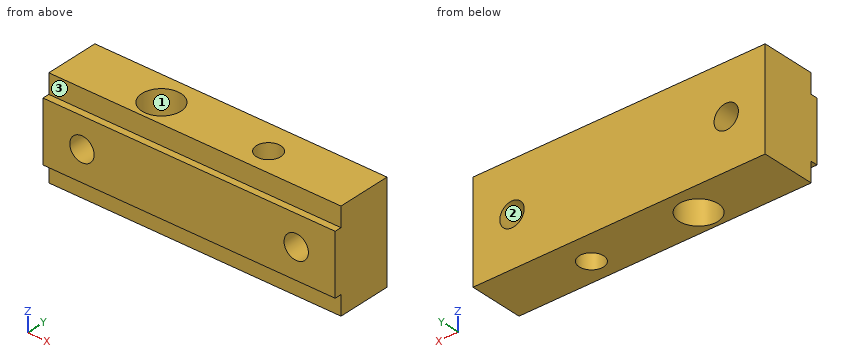
```python
from build123d import *

# Parameters (mm, degrees)
SKETCH1_W                  = 30
SKETCH1_H                  = 10.2
BOSS_EXTRUDE1_DEPTH        = 6.25
F_4_0_4_DIAMETER_HOLE1_D   = 4
F_2_5_2_5_DIAMETER_HOLE2_D = 2.5
F_2_5_2_5_DIAMETER_HOLE1_D = 2.5
SKETCH6_W                  = 2
SKETCH6_H                  = 0.7
CUT_EXTRUDE1_DEPTH         = 31


with BuildPart() as part:
    # Sketch1 → Boss-Extrude1 (new body)
    with BuildSketch(Plane(origin=(0, 0, 0), x_dir=(1, 0, 0), z_dir=(0, 1, 0))):
        with Locations((15, 5.1)):
            Rectangle(SKETCH1_W, SKETCH1_H)
    extrude(amount=BOSS_EXTRUDE1_DEPTH)

    # Ø4.0 (4) Diameter Hole1 (through all)
    with Locations(Plane.XY):
        with Locations((9.5, 3.125)):
            Hole(F_4_0_4_DIAMETER_HOLE1_D / 2)

    # Ø2.5 (2.5) Diameter Hole2 (through all)
    with Locations(Plane.XY):
        with Locations((20.5, 3.125)):
            Hole(F_2_5_2_5_DIAMETER_HOLE2_D / 2)

    # Ø2.5 (2.5) Diameter Hole1 (through all)
    with Locations(Plane(origin=(0, 6.25, 0), x_dir=(-1, 0, 0), z_dir=(0, 1, 0))):
        with Locations((-4, -5.1), (-26, -5.1)):
            Hole(F_2_5_2_5_DIAMETER_HOLE1_D / 2)

    # Sketch6 → Cut-Extrude1 (cut, through all)
    with BuildSketch(Plane(origin=(30, 0, 0), x_dir=(0, 0, -1), z_dir=(1, 0, 0))):
        with Locations((9.2, 0.35)):
            Rectangle(SKETCH6_W, SKETCH6_H)
    cut_extrude1 = extrude(amount=-CUT_EXTRUDE1_DEPTH, mode=Mode.SUBTRACT)

    # Mirror1: Cut-Extrude1 across plane
    add(cut_extrude1.mirror(Plane.XY.offset(-5.1)), mode=Mode.SUBTRACT)


solid = part.part
```
Geometry check sheet. Reference: the model listing, model coordinates, mm. Face numbers are marked on the shaded views. Give positions to 0.01 mm unless a question says otherwise; leave off trailing zeros. Loops run counter-clockwise (first coordinate to the right, second up) from the corner with the lowest first, then second, coordinate; pieces in that order, holes last. Notation, with made-up numbers: M 65,40.25 L 97,40.25 A15 cw 97,45.25 Z; hole C 35,49.5 d1. An arc over 180 degrees is marked long. Write item = value, one per line. Start each with the question number.
1. Thickness scan on probe 1 along Y at (x, z) = (20.5, -3.75) (3 decimals); probe 2 along Z at (x, y) = (26, 2.25); probe 3 along X at (y, z) = (2.75, -1.75). Record the ranges inside material, lowest first.
2. Section check C-C, the plane z = -5.1. Enter the section's corners in (x, y) (3 decimals), plus the area to 3 significant figures.
3. Go/stop test with flat-tipped pins: P1, Ø1.5, axis at x = 20.5, y = 3.125, coming from the +Z side; P2, Ø1, axis at x = 16.5, z = -9.5, coming from the -Y side. Record where each tip stops, or that it passes through.
4. Section check A-A, the plane x = 9.5. Enter the section's corners in (y, z) (3 decimals).
5. Section check B-B, the plane y = 3.5. Enter the section's corners in (x, z), plus the area to 3 significant figures.
6. Draft check along Y on the marked faces 1, 2 and 3. Enter one of: +Y half, -Y half, draft (parallel to the pull), parting line (faces both ways), or undercut.
7. Section check D-D, the plane y = 4.75. Enter the section's corners in (x, z).
Values follow:
q1.probe_1 = 0 to 1.875, 4.375 to 6.25
q1.probe_2 = -10.2 to -6.35, -3.85 to 0
q1.probe_3 = 0 to 7.54, 11.46 to 19.31, 21.69 to 30
q2.outline = M 0,0 L 2.75,0 L 2.75,6.25 L 0,6.25 Z; M 5.25,0 L 24.75,0 L 24.75,6.25 L 5.25,6.25 Z; M 27.25,0 L 30,0 L 30,6.25 L 27.25,6.25 Z; hole C 9.5,3.125 d4; hole C 20.5,3.125 d2.5
q2.area = 139 mm^2
q3.P1 = through
q3.P2 = 0.7
q4.outline = M 0,-8.2 L 0.7,-8.2 L 0.7,-10.2 L 1.125,-10.2 L 1.125,0 L 0.7,0 L 0.7,-2 L 0,-2 Z; M 5.125,-10.2 L 6.25,-10.2 L 6.25,0 L 5.125,0 Z
q5.outline = M 0,-10.2 L 7.54,-10.2 L 7.54,0 L 0,0 Z; M 11.46,-10.2 L 19.31,-10.2 L 19.31,0 L 11.46,0 Z; M 21.69,-10.2 L 30,-10.2 L 30,0 L 21.69,0 Z; hole C 4,-5.1 d2.5; hole C 26,-5.1 d2.5
q5.area = 232 mm^2
q6.face_1 = undercut
q6.face_2 = draft
q6.face_3 = -Y half
q7.outline = M 0,-10.2 L 8.33,-10.2 L 8.33,0 L 0,0 Z; M 10.67,-10.2 L 30,-10.2 L 30,0 L 10.67,0 Z; hole C 4,-5.1 d2.5; hole C 26,-5.1 d2.5
